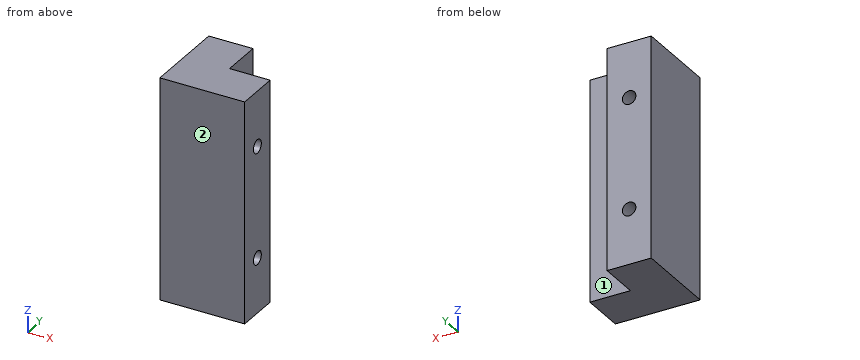
from build123d import *

# Parameters (mm, degrees)
EXTRUDE_1_DEPTH     = 24.5
SKETCH_2_R          = 0.75
CUT_EXTRUDE_1_DEPTH = 5
SKETCH_3_R          = 0.75
CUT_EXTRUDE_2_DEPTH = 5


with BuildPart() as part:
    # 草圖1 → 填料-伸長1 (new body)
    with BuildSketch(Plane.XY):
        Polygon((0, 9.4), (0, 0), (9.4, 0), (9.4, 4.9), (4.9, 4.9), (4.9, 9.4), align=None)
    extrude(amount=EXTRUDE_1_DEPTH)

    # 草圖2 → 除料-伸長1 (cut)
    with BuildSketch(Plane(origin=(9.4, 0, 0), x_dir=(0, 0, -1), z_dir=(1, 0, 0))):
        with Locations(Location((-6.1, 2.45, 0), (0, 0, 90))):
            Circle(SKETCH_2_R)
        with Locations(Location((-18.4, 2.45, 0), (0, 0, 90))):
            Circle(SKETCH_2_R)
    extrude(amount=-CUT_EXTRUDE_1_DEPTH, mode=Mode.SUBTRACT)

    # 草圖3 → 除料-伸長2 (cut)
    with BuildSketch(Plane(origin=(0, 9.4, 0), x_dir=(1, 0, 0), z_dir=(0, 1, 0))):
        with Locations(Location((2.45, -6.1, 0), (0, 0, 180))):
            Circle(SKETCH_3_R)
        with Locations(Location((2.45, -18.4, 0), (0, 0, 180))):
            Circle(SKETCH_3_R)
    extrude(amount=-CUT_EXTRUDE_2_DEPTH, mode=Mode.SUBTRACT)


solid = part.part
Verification items for the finished model (mm, model axes). Face numbers are marked on the shaded views. A direction names the side the tool comes from. Round coordinates to 2 decimals unless told otherwise and drop trailing zeros. Loops run counter-clockwise (first coordinate to the right, second up) from the corner with the lowest first, then second, coordinate; pieces in that order, holes last. Notation, with made-up numbers: (30, 73) - (56, 73) arc R20 cw to (56, 93) - close; hole circle Ø10 at (82.25, 56.5). An arc over 180 degrees is marked (long way). Use a Markdown table: item, result. Add a question column.
1. Access from +Z, -Z, +X, -X, +Y, -Y to the whole of each face (thin tool, end or side, straight path). Record for the marked faces 1 and 2.
2. Section check B-B, the plane z = 6.1. Record the boundary of the cut face in (x, y).
3. Section check D-D, the plane y = 2. Record the boundary of the cut face in (x, z), plus the area to 3 significant figures.
4. Section check A-A, the plane y = 8. Record the boundary of the cut face in (x, z), plus the area to 3 significant figures.
5. Gauge pin test, flat ends, axial feed: pin 1 (1.3 mm diameter, centred on y = 7.5, z = 16.5, fed in from +X); pin 2 (2.5 mm diameter, centred on x = 2.45, z = 18.4, fed in from -Y); pin 3 (1.3 mm diameter, centred on x = 8.5, z = 17, fed in from +Y); pin 4 (0.8 mm diameter, centred on x = 2.5, z = 6, fed in from +Y). Record the tip position at first contact, or that the pin passes through.
6. Thickness scan on probe 1 along Z at (x, y) = (6.3, 2.45); probe 2 along Y at (x, z) = (8.5, 20.25). Record the ranges inside material, lowest first. Write a range as [from, to].
7. Section check C-C, the plane x = 2.45. Record the boundary of the cut face in (y, z).
Checks:
| question | item | result |
|---|---|---|
| 1 | face 1 | +Z, -Z, +X, +Y |
| 1 | face 2 | +Z, -Z, +X, -X, -Y |
| 2 | outline | (0, 0) - (9.4, 0) - (9.4, 1.7) - (4.4, 1.7) - (4.4, 3.2) - (9.4, 3.2) - (9.4, 4.9) - (4.9, 4.9) - (4.9, 9.4) - (3.2, 9.4) - (3.2, 4.4) - (1.7, 4.4) - (1.7, 9.4) - (0, 9.4) - close |
| 3 | outline | (0, 0) - (9.4, 0) - (9.4, 5.5) - (4.4, 5.5) - (4.4, 6.7) - (9.4, 6.7) - (9.4, 17.8) - (4.4, 17.8) - (4.4, 19) - (9.4, 19) - (9.4, 24.5) - (0, 24.5) - close |
| 3 | area | 218 mm^2 |
| 4 | outline | (0, 0) - (4.9, 0) - (4.9, 24.5) - (0, 24.5) - close; hole circle Ø1.5 at (2.45, 6.1); hole circle Ø1.5 at (2.45, 18.4) |
| 4 | area | 117 mm^2 |
| 5 | pin 1 | stops at x = 4.9 |
| 5 | pin 2 | stops at y = 0 |
| 5 | pin 3 | stops at y = 4.9 |
| 5 | pin 4 | stops at y = 4.4 |
| 6 | probe 1 | z = [0, 5.35], [6.85, 17.65], [19.15, 24.5] |
| 6 | probe 2 | y = [0, 4.9] |
| 7 | outline | (0, 0) - (9.4, 0) - (9.4, 5.35) - (4.4, 5.35) - (4.4, 6.85) - (9.4, 6.85) - (9.4, 17.65) - (4.4, 17.65) - (4.4, 19.15) - (9.4, 19.15) - (9.4, 24.5) - (0, 24.5) - close |
